Source: CAD feature listing. Evaluate the final solid. Frame: model axes, mm. Give positions to 0.01 mm unless a question says otherwise; leave off trailing zeros. Write each loop counter-clockwise with the first axis right and the second up, starting at its lowest first coordinate (ties: lowest second). Pieces come first, ordered by that corner, then holes. Notation, with made-up numbers: (-21.5, 50) - (0.5, 50) arc R11 ccw to (0.5, 66) - close; hole circle Ø1 at (58, -13.75). An arc over 180 degrees is marked (long way). Answer as a JSON object with one key per item and string values. Group by question number.
Autodesk Inventor part; units mm, degrees
ref_plane "YZ Plane" through (0, 0, 0) normal (1, 0, 0) x (0, 1, 0)
ref_plane "XZ Plane" through (0, 0, 0) normal (0, 1, 0) x (-1, 0, 0)
ref_plane "XY Plane" through (0, 0, 0) normal (0, 0, 1) x (1, 0, 0)
sketch "Sketch1" plane through (0, 0, 0) normal (0, 1, 0) x (-1, 0, 0)
  circle A0 centre (-16.9706, -0.5878) radius 1.5
  circle A1 centre (16.9706, -0.5878) radius 1.5
  circle A2 centre (30, -5.1319) radius 1.5
  circle A3 centre (-30, -5.1319) radius 1.5
  circle A4 centre (16.9706, -0.5878) radius 5 construction
  circle A5 centre (-16.9706, -0.5878) radius 5 construction
  arc A6 (-31.1155, 2.2846) -> (-30, -12.6319) centre (-30, -5.1319) ccw
  arc A7 (30, -12.6319) -> (31.1155, 2.2846) centre (30, -5.1319) ccw
  line L0 (30, -12.6319) -> (-30, -12.6319)
  line L1 (-16.9706, 4.4122) -> (16.9706, 4.4122)
  line L2 (-16.9706, 4.4122) -> (-31.1155, 2.2846)
  line L3 (16.9706, 4.4122) -> (31.1155, 2.2846)
  arc A8 (31.1155, 2.2846) -> (23.1456, -2.0878) centre (30, -5.1319) ccw
  arc A9 (-30, -12.6319) -> (-23.1456, -2.0878) centre (-30, -5.1319) ccw construction
  line L4 (0, 4.2106) -> (0, -4.2106) construction
  line L5 (0, -4.2106) -> (3.1574, -4.2106) construction
  line L6 (0, -4.2106) -> (0, -12.6319) construction
  circle A10 centre (0, 0) radius 1.55
  line L7 (0, -8.4213) -> (15.6117, -8.4213) construction
  line L8 (0, -8.4213) -> (-15.6117, -8.4213) construction
  circle A11 centre (7.8058, -8.4213) radius 1.55 construction
  circle A12 centre (-7.8058, -8.4213) radius 1.55 construction
  line L9 (16.9706, -2.0878) -> (-16.9706, -2.0878)
  line L10 (16.9706, -2.0878) -> (23.1456, -2.0878)
  line L11 (-16.9706, -2.0878) -> (-23.1456, -2.0878)
  arc A13 (-23.1456, -2.0878) -> (-31.1155, 2.2846) centre (-30, -5.1319) ccw
  arc A14 (23.1456, -2.0878) -> (30, -12.6319) centre (30, -5.1319) ccw construction
  line L12 (7.8058, -12.6319) -> (7.8058, -2.0878) construction
  line L13 (-7.8058, -12.6319) -> (-7.8058, -2.0878) construction
  line L14 (3.5375, -12.6319) -> (3.5375, -2.0878) construction
  line L15 (3.5375, -7.3599) -> (10.9646, -7.3599) construction
  line L16 (3.5375, -7.3599) -> (-12.9158, -7.3599) construction
  circle A15 centre (7.8058, -7.3599) radius 1.55
  circle A16 centre (-7.8058, -7.3599) radius 1.55
  circle A17 centre (-16.9706, -0.5878) radius 3.25
  circle A18 centre (16.9706, -0.5878) radius 3.25
  circle A19 centre (16.9706, -0.5878) radius 2.75 construction
  line L17 (15.3828, -3.3378) -> (13.7951, -0.5878) construction
  line L18 (13.7951, -0.5878) -> (15.3828, 2.1622) construction
  line L19 (15.3828, 2.1622) -> (18.5583, 2.1622) construction
  line L20 (18.5583, 2.1622) -> (20.146, -0.5878) construction
  line L21 (20.146, -0.5878) -> (18.5583, -3.3378) construction
  line L22 (18.5583, -3.3378) -> (15.3828, -3.3378) construction
  point P0 (0, 0)
  point P1 (19.8537, -2.0878)
  point P2 (14.0874, -2.0878)
  point P3 (-14.0874, -2.0878)
  point P4 (-19.8537, -2.0878)
  point P5 (16.9706, -3.3378)
  dimension "d0" = 10
  dimension "d1" = 10
  dimension "d20" = 5.5
  dimension "d2" = 15
  dimension "d3" = 15
  dimension "d4" = 3.1
  dimension "d5" = 3.1
  dimension "d6" = 3.1
  dimension "d13" = 10.5442
  dimension "d14" = 3.1
  dimension "d15" = 3.1
  dimension "d16" = 6.5
  dimension "d17" = 6.5
extrude "Extrusion1" add sketch "Sketch1" along normal blind 3 contours L9 A18 L10 A8 A7 L0 A6 A13 L11 A17
fillet "Fillet2" radius 3 4 edges at (-19.8537, 1.5, -2.0878) (-14.0874, 1.5, -2.0878) (14.0874, 1.5, -2.0878) (19.8537, 1.5, -2.0878)
fillet "Fillet3" radius 4 2 edges at (-23.1456, 1.5, -2.0878) (23.1456, 1.5, -2.0878)
properties part number "prig to kauri conversion plate"
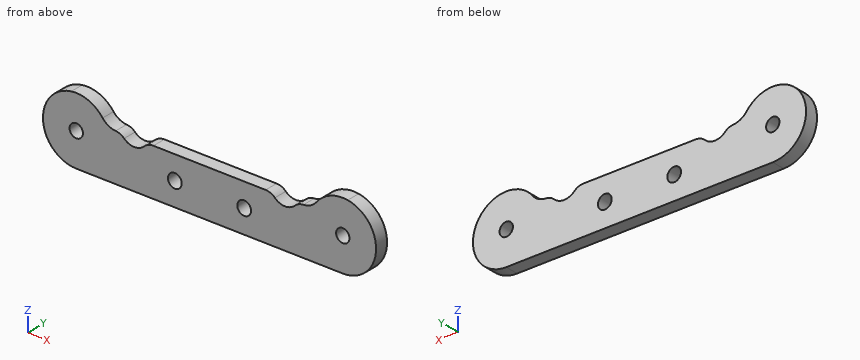
Q1. First-contact query: pin 1 Ø0.9 at (x, y) = (-3.5, 1.5) entering from +Z. Flat tip, straight axial feed; report the tip coordinate or a pass-through.
Q2. Ray query, probe 1 along Z at (x, y) = (30, 0.6); probe 2 along X at (y, z) = (1.65, -5.5); probe 3 along X at (y, z) = (2.3, -7.75). Return the intervals inside material, ascending. Write a range as [from, to].
Q3. Section D-D on x = 1. Return the cut outline in (y, z), then the cut area to 3 significant figures.
Q4. Section A-A on z = -4.5. Return the cut outline in (x, y).
Q5. Section C-C on x = -20. Return the cut outline in (y, z), then the cut area to 3 significant figures.
Q6. Section B-B on y = 0.55. State how many separate pieces and enclosed holes the cut face has, then the cut area to 3 significant figures.
Taken from the geometry:
{
 "1": {"pin 1": "stops at z = -2.09"},
 "2": {"probe 1": "z = [-12.63, -6.63], [-3.63, 2.37]", "probe 2": "x = [-37.49, -31.45], [-28.55, 28.55], [31.45, 37.49]", "probe 3": "x = [-37.03, -9.31], [-6.31, 6.31], [9.31, 37.03]"},
 "3": {"outline": "(0, -12.63) - (3, -12.63) - (3, -2.09) - (0, -2.09) - close", "area": "31.6 mm²"},
 "4": {"outline": "(-37.47, 0) - (-31.36, 0) - (-31.36, 3) - (-37.47, 3) - close; (-28.64, 0) - (28.64, 0) - (28.64, 3) - (-28.64, 3) - close; (31.36, 0) - (37.47, 0) - (37.47, 3) - (31.36, 3) - close"},
 "5": {"outline": "(0, -12.63) - (3, -12.63) - (3, -2.39) - (0, -2.39) - close", "area": "30.7 mm²"},
 "6": {"separate pieces": "1", "enclosed holes": "4", "area": "810 mm²"}
}
